from build123d import *

# Parameters (mm, degrees)
BOX017_W          = 18
BOX017_H          = 18
BOX017_DEPTH      = 36
CYLINDER010_R     = 1
CYLINDER010_DEPTH = 70
BOX015_W          = 18
BOX015_H          = 18
BOX015_DEPTH      = 6
ARRAY007_Z_COUNT  = 2
ARRAY007_Z_PITCH  = 36
BOX016_W          = 18
BOX016_H          = 18
BOX016_DEPTH      = 36
BOX014_W          = 18
BOX014_H          = 18
BOX014_DEPTH      = 42
FILLET001_R       = 7


with BuildPart() as cube017:
    # Box017 → Box017 (new body)
    with BuildSketch(Plane(origin=(-2, 14, 3), x_dir=(1, 0, 0), z_dir=(0, 0, 1))):
        with Locations((9, 9)):
            Rectangle(BOX017_W, BOX017_H)
    extrude(amount=BOX017_DEPTH)


with BuildPart() as cylinder010:
    # Cylinder010 → Cylinder010 (new body)
    with BuildSketch(Plane(origin=(9, 9, -17), x_dir=(1, 0, 0), z_dir=(0, 0, 1))):
        Circle(CYLINDER010_R)
    extrude(amount=CYLINDER010_DEPTH)


with BuildPart() as array007:
    # Box015 → Box015 (new body)
    with BuildSketch(Plane(origin=(-5, 5, 0), x_dir=(1, 0, 0), z_dir=(0, 0, 1))):
        with Locations((9, 9)):
            Rectangle(BOX015_W, BOX015_H)
    extrude(amount=BOX015_DEPTH)

    # Array007 Z: Array007 ×2


with BuildPart() as array007_1:
    add(array007.part)
    with Locations(*[(0, 0, i * ARRAY007_Z_PITCH) for i in range(1, ARRAY007_Z_COUNT)]):
        add(array007.part)


with BuildPart() as cone002:
    # Cone002 → Cone002 (revolve)
    with BuildSketch(Plane(origin=(9, 9, 0), x_dir=(1, 0, 0), z_dir=(0, -1, 0))):
        Polygon((0, 0), (2.9, 0), (1.5, 3.5), (0, 3.5), align=None)
    revolve(axis=Axis((9, 9, 0), (0, 0, 1)))


with BuildPart() as cone003:
    # Cone003 → Cone003 (revolve)
    with BuildSketch(Plane(origin=(9, 9, 38.5), x_dir=(1, 0, 0), z_dir=(0, -1, 0))):
        Polygon((0, 0), (1.5, 0), (2.9, 3.5), (0, 3.5), align=None)
    revolve(axis=Axis((9, 9, 38.5), (0, 0, 1)))


with BuildPart() as fusion006:
    # Box016 → Box016 (new body)
    with BuildSketch(Plane(origin=(-14, 2, 3), x_dir=(1, 0, 0), z_dir=(0, 0, 1))):
        with Locations((9, 9)):
            Rectangle(BOX016_W, BOX016_H)
    extrude(amount=BOX016_DEPTH)

    # Fusion006: union Cube017, Cylinder010, Array007, Cone002, Cone003
    add(cube017.part)
    add(cylinder010.part)
    add(array007_1.part)
    add(cone002.part)
    add(cone003.part)


with BuildPart() as fillet001:
    # Box014 → Box014 (new body)
    with BuildSketch(Plane.XY):
        with Locations((9, 9)):
            Rectangle(BOX014_W, BOX014_H)
    extrude(amount=BOX014_DEPTH)

    # Cut007: cut Fusion006
    add(fusion006.part, mode=Mode.SUBTRACT)

    # Fillet001
    fillet001_edges = [fillet001.edges().sort_by_distance(p)[0] for p in [
        (4, 14, 21),
    ]]
    fillet(fillet001_edges, radius=FILLET001_R)


solid = fillet001.part
Geometry check sheet. Reference: the model listing, model coordinates, mm. A direction names the side the tool comes from. Give positions to 0.01 mm unless a question says otherwise; leave off trailing zeros. Loops run counter-clockwise (first coordinate to the right, second up) from the corner with the lowest first, then second, coordinate; pieces in that order, holes last.
(1) Section check D-D on x = 9. Record the cut outline in (y, z), then the cut area to 3 significant figures.
From the geometry:
outline: (0, 0) - (5, 0) - (5, 6) - (8, 6) - (8, 36) - (5, 36) - (5, 42) - (0, 42) - close; (10, 6) - (13.71, 6) - (13.71, 36) - (10, 36) - close
area: 411 mm2
(2) Section check B-B on z = 18. Record the cut outline in (x, y), then the cut area to 3 significant figures.
From the geometry:
outline: (0, 0) - (18, 0) - (18, 18) - (16, 18) - (16, 14) - (11, 14) arc R7 ccw to (4, 7) - (4, 2) - (0, 2) - close; hole circle Ø2 at (9, 9)
area: 198 mm2
(3) Section check C-C on y = 9. Record the cut outline in (x, z).
From the geometry:
outline: (4.29, 6) - (8, 6) - (8, 36) - (4.29, 36) - close; (10, 6) - (13, 6) - (13, 0) - (18, 0) - (18, 42) - (13, 42) - (13, 36) - (10, 36) - close
(4) Release check for a two-part mould opening along Z. For faces 5 (the flat face through (15, 5, 0)), 6 (the flat face through (17, 18, 21)), 7 (the flat face through (2, 4, 3)) record: released by +Z, released by -Z, zero draft, split by the parting line, or undercut.
From the geometry:
face 5: released by -Z
face 6: zero draft
face 7: undercut
(5) Set-up check for faces 1 (the flat face through (8, 11, 6)), 2 (the flat face through (8, 5, 39)), 3 (the flat face through (4, 4, 21)), 4 (the flat face through (0, 1, 21)): record each of +Z, -Z, +X, -X, +Y, -Y from which the full face is reachable in a straight line by a thin tool's end or side.
From the geometry:
face 1: -Z, -X, +Y
face 2: +Z, -X, +Y
face 3: -X, +Y
face 4: +Z, -Z, -X, +Y, -Y
(6) Section check A-A on x = 14.5. Record the cut outline in (y, z).
From the geometry:
outline: (0, 0) - (18, 0) - (18, 3) - (14, 3) - (14, 39) - (18, 39) - (18, 42) - (0, 42) - close
(7) Thickness scan on L1, parallel to Y at x = 11.25, z = 8; L2, parallel to X at y = 14.5, z = 28; L3, parallel to Z at x = 9, y = 13.25. Record the ranges inside material, lowest first.
From the geometry:
L1: y = 0 to 14
L2: x = 16 to 18
L3: z = 6 to 36
(8) Depth check by flat-ended pin: pin 1 Ø8 at (y, z) = (13.5, 5.5) entering from -X; pin 2 Ø1.8 at (x, z) = (6.5, 39) entering from +Y; pin 3 Ø10 at (x, z) = (8.5, 19.5) entering from +Y. Enter the tip coordinate at first touch or a pass-through.
From the geometry:
pin 1: stops at x = 4.47
pin 2: stops at y = 5
pin 3: stops at y = 14
